from build123d import *

# Parameters (mm, degrees)
ESQUISSE1_W              = 30
ESQUISSE1_H              = 30
BOSS_EXTRU_1_DEPTH       = 30
ESQUISSE2_W              = 13
ESQUISSE2_H              = 15
ENL_V_MAT_EXTRU_1_DEPTH  = 6
ESQUISSE3_W              = 3.5
ESQUISSE3_H              = 15
ENL_V_MAT_EXTRU_2_DEPTH  = 3
ESQUISSE4_R              = 2.5
ENL_V_MAT_EXTRU_18_DEPTH = 52.961524227
CONG_1_R                 = 3


with BuildPart() as part:
    # Esquisse1 → Boss.-Extru.1 (new body)
    with BuildSketch(Plane.XY):
        with Locations((-15, -15)):
            Rectangle(ESQUISSE1_W, ESQUISSE1_H)
    extrude(amount=BOSS_EXTRU_1_DEPTH)

    # Esquisse2 → Enlèv. mat.-Extru.1 (cut)
    with BuildSketch(Plane(origin=(0, 0, 0), x_dir=(-1, 0, 0), z_dir=(0, 0, -1))):
        with Locations((15, -7.5)):
            Rectangle(ESQUISSE2_W, ESQUISSE2_H)
    extrude(amount=-ENL_V_MAT_EXTRU_1_DEPTH, mode=Mode.SUBTRACT)

    # Esquisse3 → Enlèv. mat.-Extru.2 (cut)
    with BuildSketch(Plane(origin=(0, 0, 0), x_dir=(-1, 0, 0), z_dir=(0, 0, -1))):
        with Locations((19.75, -22.5)):
            Rectangle(ESQUISSE3_W, ESQUISSE3_H)
    extrude(amount=-ENL_V_MAT_EXTRU_2_DEPTH, mode=Mode.SUBTRACT)

    # Esquisse4 → Enlèv. mat.-Extru.18 (cut, through all)
    with BuildSketch(Plane(origin=(0, 0, 0), x_dir=(-1, 0, 0), z_dir=(0, 0, -1))):
        with Locations((14, -21.038960512)):
            Circle(ESQUISSE4_R)
    extrude(amount=-ENL_V_MAT_EXTRU_18_DEPTH, mode=Mode.SUBTRACT)

    # Congé1
    cong_1_edges = [part.edges().sort_by_distance(p)[0] for p in [
        (-30, -15, 0),
        (0, -15, 0),
        (0, -30, 15),
        (-30, -30, 15),
        (-30, 0, 15),
        (0, 0, 15),
    ]]
    fillet(cong_1_edges, radius=CONG_1_R)


solid = part.part
The model under review builds one solid part; all positions refer to its coordinate system, in mm. A direction names the side the tool comes from. Give positions to 0.01 mm unless a question says otherwise; leave off trailing zeros. Order: outer loops, then holes, each group sorted by start corner. A loop starts at its lowest first (then second) coordinate and runs counter-clockwise, first axis right, second up. Notation, with made-up numbers: M -10.5,14.25 L 9.5,14.25 A15 ccw 9.5,18.25 Z; hole C 58,-4 d2. An arc over 180 degrees is marked long. Answer in a Markdown table with one row per item. Add a question column.
1. To check wall thickness, follow line 1 along Y through (x, z) = (-14, 9.5); line 2 along X through (y, z) = (-4.75, 5.25); line 3 along Z through (x, y) = (-16.5, -6.75). State the ranges of each line that lie inside material, in increasing order.
2. Mouldability with a two-part tool opening along X and no side actions: class faces 1 (the flat face through (-15, -15, 30)), 2 (the cylindrical face through (-0.9, -14.79, 0.86)), 3 (the flat face through (-21.5, -12, 2)) as released by +X, released by -X, zero draft, split by the parting line, or undercut.
3. Add section C-C on y = -19.25. State the section outline as (x, z) points, plus the area to 3 significant figures.
4. For pin 1 Ø0.9 at (y, z) = (-20.5, 1) entering from -X; pin 2 Ø1.8 at (x, z) = (-14, 4.5) entering from +Y, all flat-tipped, find the tip position at first contact; note any pin that passes through.
5. Add section B-B on z = 2.25. State the section outline as (x, y) points.
6. Add section A-A on x = -14. State the section outline as (y, z) points, plus the area to 3 significant figures.
7. Add section D-D on z = 26. State the section outline as (x, y) points.
8. Machinability: for faces 4 (the cylindrical face through (-29.14, -14.79, 0.9)), 5 (the flat face through (-18, -23, 1)), 6 (the flat face through (-15, -15, 3)), which of the approach directions +Z, -Z, +X, -X, +Y, -Y give a long, thin tool a straight path to every point of the face, cutting with its end or side? Answer none if there is none.
The answers:
| question | item | result |
|---|---|---|
| 1 | line 1 | -30 to -23.54, -18.54 to 0 |
| 1 | line 2 | -30 to -21.5, -8.5 to 0 |
| 1 | line 3 | 6 to 30 |
| 2 | face 1 | zero draft |
| 2 | face 2 | released by +X |
| 2 | face 3 | undercut |
| 3 | outline | M -30,3 A3 ccw -27,0 L -21.5,0 L -21.5,3 L -18,3 L -18,0 L -15.75,0 L -15.75,30 L -30,30 Z; M -12.25,0 L -3,0 A3 ccw 0,3 L 0,30 L -12.25,30 Z |
| 3 | area | 781 mm2 |
| 4 | pin 1 | x = -29.57 |
| 4 | pin 2 | y = -15 |
| 5 | outline | M -29.9,-27.75 A3 ccw -27,-30 L -21.5,-30 L -21.5,0 L -27,0 A3 ccw -29.9,-2.25 Z; M -18,-30 L -3,-30 A3 ccw -0.1,-27.75 L -0.1,-2.25 A3 ccw -3,0 L -8.5,0 L -8.5,-15 L -18,-15 Z; hole C -14,-21.04 d5 |
| 6 | outline | M -30,0 L -23.54,0 L -23.54,30 L -30,30 Z; M -18.54,0 L -15,0 L -15,6 L 0,6 L 0,30 L -18.54,30 Z |
| 6 | area | 660 mm2 |
| 7 | outline | M -30,-27 A3 ccw -27,-30 L -3,-30 A3 ccw 0,-27 L 0,-3 A3 ccw -3,0 L -27,0 A3 ccw -30,-3 Z; hole C -14,-21.04 d5 |
| 8 | face 4 | -Z, -X, +Y, -Y |
| 8 | face 5 | -Z, +Y, -Y |
| 8 | face 6 | -Z, +Y |
